from build123d import *

# Parameters (mm, degrees)
SKETCH_1_W          = 2.5
SKETCH_1_H          = 103
SKETCH_1_W_2        = 2
SKETCH_1_H_2        = 95
EXTRUDE_1_DEPTH     = 99.5
CUT_EXTRUDE_2_DEPTH = 4.5
CUT_EXTRUDE_3_DEPTH = 58.5
CUT_EXTRUDE_4_DEPTH = 4.5
SKETCH_6_W          = 1.6
SKETCH_6_H          = 17
CUT_EXTRUDE_5_DEPTH = 10
SKETCH_7_R          = 0.5
EXTRUDE_2_DEPTH     = 9.886463591


with BuildPart() as part:
    # 스케치1 → 보스-돌출1 (new body)
    with BuildSketch(Plane(origin=(0, 0, 0), x_dir=(1, 0, 0), z_dir=(0, 1, 0))):
        with Locations((1.25, -51.5)):
            Rectangle(SKETCH_1_W, SKETCH_1_H)
        with Locations((3.5, -51.5)):
            Rectangle(SKETCH_1_W_2, SKETCH_1_H_2)
    extrude(amount=EXTRUDE_1_DEPTH)

    # 스케치2 → 컷-돌출2 (cut)
    with BuildSketch(Plane(origin=(4.5, 0, 0), x_dir=(0, 0, -1), z_dir=(1, 0, 0))):
        with BuildLine():
            Line((-62, 10), (-62, 0))
            Line((-62, 0), (-41, 0))
            Line((-41, 0), (-41, 10))
            ThreePointArc((-41, 10), (-51.5, 20.5), (-62, 10))
        make_face()
    extrude(amount=-CUT_EXTRUDE_2_DEPTH, mode=Mode.SUBTRACT)

    # 스케치3 → 컷-돌출3 (cut)
    with BuildSketch(Plane(origin=(0, 99.5, 0), x_dir=(1, 0, 0), z_dir=(0, 1, 0))):
        Polygon((2.5, -4), (2.5, 0), (0, 0), (0, -103), (2.5, -103), (2.5, -99), (4.5, -99), (4.5, -4), align=None)
    extrude(amount=-CUT_EXTRUDE_3_DEPTH, mode=Mode.SUBTRACT)

    # 스케치4 → 컷-돌출4 (cut)
    with BuildSketch(Plane(origin=(0, 41, 0), x_dir=(1, 0, 0), z_dir=(0, 1, 0))):
        Polygon((4.5, -4), (2.5, -4), (2.5, 0), (0, 0), (0, -103), (2.5, -103), (2.5, -99), (4.5, -99), align=None)
    extrude(amount=-CUT_EXTRUDE_4_DEPTH, mode=Mode.SUBTRACT)

    # 스케치6 → 컷-돌출5 (cut)
    with BuildSketch(Plane.XZ):
        with Locations((0.8, 74)):
            Rectangle(SKETCH_6_W, SKETCH_6_H)
    extrude(amount=-CUT_EXTRUDE_5_DEPTH, mode=Mode.SUBTRACT)

    # 스케치7 → 보스-돌출2 (add)
    with BuildSketch(Plane.XY.offset(103)):
        with Locations(Location((1.25, 34.722848579, 0), (0, 0, 180))):
            Circle(SKETCH_7_R)
        with Locations(Location((1.25, 24.722848579, 0), (0, 0, 180))):
            Circle(SKETCH_7_R)
        with Locations(Location((1.25, 14.722848579, 0), (0, 0, 180))):
            Circle(SKETCH_7_R)
        with Locations(Location((1.25, 4.722848579, 0), (0, 0, 180))):
            Circle(SKETCH_7_R)
    extrude(amount=EXTRUDE_2_DEPTH)


solid = part.part
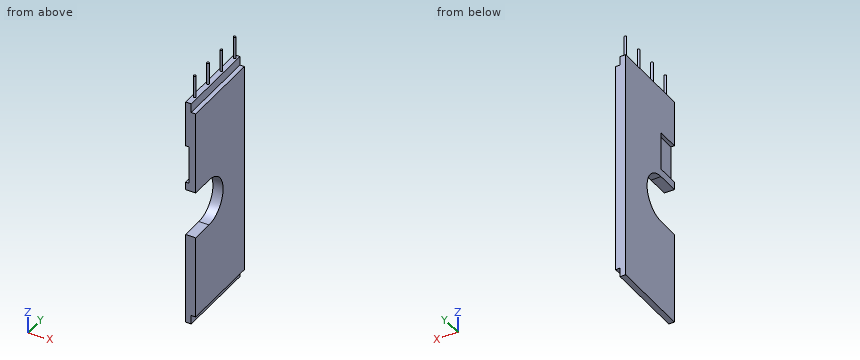
Can you work these out from the model? Positions are in its coordinate system, mm. Round coordinates to 2 decimals unless told otherwise and drop trailing zeros. Loops run counter-clockwise (first coordinate to the right, second up) from the corner with the lowest first, then second, coordinate; pieces in that order, holes last. Notation, with made-up numbers: (81.25, 42) - (110.25, 42) arc R20 cw to (110.25, 51) - close; hole circle Ø11 at (-33, 45). An arc over 180 degrees is marked (long way). Write item = value, one per line. Start each with the question number.
(1) For P1, Ø0.8, axis at x = 1, z = 75, coming from the -Y side; P2, Ø3, axis at y = 14, z = 1.5, coming from the +X side; P3, Ø2, axis at x = 4, y = 5, coming from the +Z side, each with a flat end and sliding along its axis, tell me the tip position at first contact or that it passes through.
(2) If we section it at B-B (y = 31.5): Please give me the cut outline in (x, z), and give its area (4 significant figures).
(3) If we section it at A-A (y = 19): Please give me the cut outline in (x, z), and give its area (3 significant figures).
(4) If I drill on probe 1 along Z at (x, y) = (0.35, 7); probe 2 along Z at (x, y) = (2.35, 5); probe 3 along Z at (x, y) = (0.4, 24), over which ranges is the centre line in solid material (lowest first)? Write a range as [from, to].
(5) If we section it at C-C (z = 51.5): Please give me the cut outline in (x, y).
Ans:
q1.P1 = 10
q1.P2 = 2.5
q1.P3 = 99
q2.outline = (0, 0) - (2.5, 0) - (2.5, 4) - (4.5, 4) - (4.5, 99) - (2.5, 99) - (2.5, 103) - (0, 103) - close
q2.area = 447.5 mm²
q3.outline = (0, 0) - (2.5, 0) - (2.5, 4) - (4.5, 4) - (4.5, 46.09) - (0, 46.09) - close; (0, 56.91) - (4.5, 56.91) - (4.5, 99) - (2.5, 99) - (2.5, 103) - (0, 103) - close
q3.area = 399 mm²
q4.probe_1 = [0, 41], [62, 65.5], [82.5, 103]
q4.probe_2 = [0, 41], [62, 103]
q4.probe_3 = [0, 103]
q5.outline = (0, 20.5) - (4.5, 20.5) - (4.5, 36.5) - (0, 36.5) - close
